Part model, mm, in its own coordinate system. Round coordinates to 2 decimals unless told otherwise and drop trailing zeros. Write each loop counter-clockwise with the first axis right and the second up, starting at its lowest first coordinate (ties: lowest second). Pieces come first, ordered by that corner, then holes.
```python
from build123d import *

# Parameters (mm, degrees)
SKETCH2_W           = 63
SKETCH2_H           = 43
BOSS_EXTRUDE1_DEPTH = 3
SKETCH3_R           = 1.5
CUT_EXTRUDE1_DEPTH  = 3
SKETCH4_R           = 1.5
CUT_EXTRUDE2_DEPTH  = 3
SKETCH5_W           = 15
SKETCH5_H           = 15
CUT_EXTRUDE3_DEPTH  = 3


with BuildPart() as part:
    # Sketch2 → Boss-Extrude1 (new body)
    with BuildSketch(Plane(origin=(0, 0, 0), x_dir=(1, 0, 0), z_dir=(0, 1, 0))):
        with Locations((-0.384353741, 1.170068027)):
            Rectangle(SKETCH2_W, SKETCH2_H)
    extrude(amount=BOSS_EXTRUDE1_DEPTH)

    # Sketch3 → Cut-Extrude1 (cut)
    with BuildSketch(Plane(origin=(0, 3, 0), x_dir=(1, 0, 0), z_dir=(0, 1, 0))):
        with Locations((28.115646259, 19.670068027)):
            Circle(SKETCH3_R)
    extrude(amount=-CUT_EXTRUDE1_DEPTH, mode=Mode.SUBTRACT)

    # Sketch4 → Cut-Extrude2 (cut)
    with BuildSketch(Plane(origin=(0, 3, 0), x_dir=(1, 0, 0), z_dir=(0, 1, 0))):
        with Locations((-28.884353741, -17.329931973)):
            Circle(SKETCH4_R)
    extrude(amount=-CUT_EXTRUDE2_DEPTH, mode=Mode.SUBTRACT)

    # Sketch5 → Cut-Extrude3 (cut)
    with BuildSketch(Plane(origin=(0, 3, 0), x_dir=(1, 0, 0), z_dir=(0, 1, 0))):
        with Locations((17.615646259, 4.170068027)):
            Rectangle(SKETCH5_W, SKETCH5_H)
    extrude(amount=-CUT_EXTRUDE3_DEPTH, mode=Mode.SUBTRACT)


solid = part.part
```
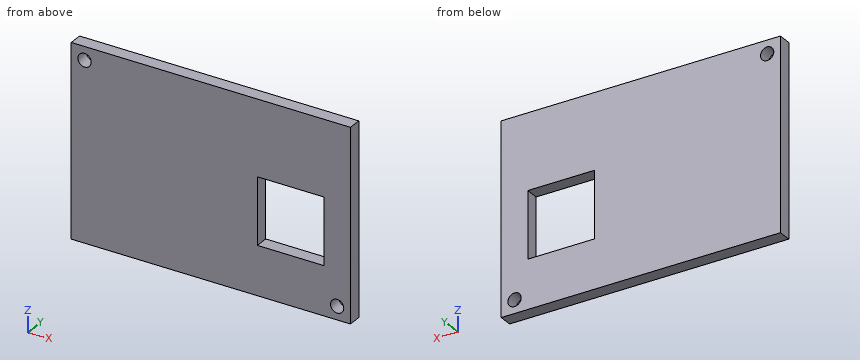
Q1. Cut at C-C on y = 2.2. Write the cut outline in (x, z), plus the area to 3 significant figures.
Values follow:
outline: (-31.88, -22.67) - (31.12, -22.67) - (31.12, 20.33) - (-31.88, 20.33) - close; hole circle Ø3 at (-28.88, 17.33); hole (10.12, -11.67) - (25.12, -11.67) - (25.12, 3.33) - (10.12, 3.33) - close; hole circle Ø3 at (28.12, -19.67)
area: 2,470 mm2
Q2. Cut at B-B on z = -10. Write the cut outline in (x, y), plus the area to 3 significant figures.
Values follow:
outline: (-31.88, 0) - (10.12, 0) - (10.12, 3) - (-31.88, 3) - close; (25.12, 0) - (31.12, 0) - (31.12, 3) - (25.12, 3) - close
area: 144 mm2
Q3. Wall check: L1, parallel to Z at x = 12, y = 1.65; L2, parallel to X at y = 1.3, z = -6.5; L3, parallel to X at y = 1.75, z = 17. Give the ranges that are in metal, low to high.
Values follow:
L1: z = -22.67 to -11.67, 3.33 to 20.33
L2: x = -31.88 to 10.12, 25.12 to 31.12
L3: x = -31.88 to -30.35, -27.42 to 31.12
Q4. Drop a flat-ended pin along its axis: pin 1 (4 mm diameter, centred on x = 13.5, z = -4.5, fed in from +Y). Give the stop position or say it passes through.
Values follow:
pin 1: passes through
Q5. Cut at A-A on x = 16.5. Write the cut outline in (y, z), plus the area to 3 significant figures.
Values follow:
outline: (0, -22.67) - (3, -22.67) - (3, -11.67) - (0, -11.67) - close; (0, 3.33) - (3, 3.33) - (3, 20.33) - (0, 20.33) - close
area: 84.0 mm2
